Model file for the job. Use its own axes, mm. A direction names the side the tool comes from. Round coordinates to 2 decimals unless told otherwise and drop trailing zeros. Write each loop counter-clockwise with the first axis right and the second up, starting at its lowest first coordinate (ties: lowest second). Pieces come first, ordered by that corner, then holes.
```python
from build123d import *

# Parameters (mm, degrees)
F0_R     = 3.9
F1_DEPTH = 25
F0_R_2   = 6
F2_DEPTH = 5
F3_SIZE2 = 3
F3_SIZE  = 0.3


with BuildPart() as f1:
    # F0 (on Front) → F1 (new body)
    with BuildSketch(Plane.XZ):
        Circle(F0_R)
    extrude(amount=F1_DEPTH)

    # F0 (on Front) → F2 (join)
    with BuildSketch(Plane.XZ):
        Circle(F0_R_2)
        Circle(F0_R, mode=Mode.SUBTRACT)
    extrude(amount=F2_DEPTH)

    # F3
    f3_edges = [f1.edges().sort_by_distance(p)[0] for p in [
        (-3.9, -25, 0),
    ]]
    f3_side = f1.faces().sort_by_distance((0, -25, 0))[0]
    chamfer(f3_edges, length=F3_SIZE, length2=F3_SIZE2, reference=f3_side)


solid = f1.part
```
1) Cut at A-A on x = 0. List the corners of the cut face in (y, z), and give its area (3 significant figures).
2) Wall check: probe 1 along Y at (x, z) = (4.25, 3.5); probe 2 along X at (y, z) = (-4.25, 0.25); probe 3 along Z at (x, y) = (-2.25, -5.5). Give the ranges that are in metal, low to high.
3) Cut at B-B on z = 0. List the corners of the cut face in (x, y), and give its area (3 significant figures).
4) Cut at C-C on y = -16.5. List the corners of the cut face in (x, z).
5) Flat gauge pins, fed straight in: pin 1 Ø3 at (x, y) = (0, -12) entering from -Z; pin 2 Ø3 at (x, y) = (-4.5, -19) entering from -Z; pin 3 Ø2 at (x, y) = (-2, -14) entering from -Z. Where does each tip first touch, or does it go through?
6) Which spindle directions (+Z, -Z, +X, -X, +Y, -Y) get a long thin tool onto all of the face, cutting with end or side? Do faces 1 (the face through (0, 0, 0)), 2 (the face through (-2.87, -13.38, 2.64)). Say none if no direction does.
7) Cut at D-D on y = -3.5. List the corners of the cut face in (x, z), and give its area (3 significant figures).
Result sheet:
1. outline: (-25, -3.6) - (-22, -3.9) - (-5, -3.9) - (-5, -6) - (0, -6) - (0, 6) - (-5, 6) - (-5, 3.9) - (-22, 3.9) - (-25, 3.6) - close
1. area: 215 mm2
2. probe 1: y = -5 to 0
2. probe 2: x = -5.99 to 5.99
2. probe 3: z = -3.19 to 3.19
3. outline: (-6, -5) - (-3.9, -5) - (-3.9, -22) - (-3.6, -25) - (3.6, -25) - (3.9, -22) - (3.9, -5) - (6, -5) - (6, 0) - (-6, 0) - close
3. area: 215 mm2
4. outline: circle Ø7.8 at (0, 0)
5. pin 1: stops at z = -3.9
5. pin 2: stops at z = -2.49
5. pin 3: stops at z = -3.77
6. face 1: +Z, -Z, +X, -X, +Y
6. face 2: -Y
7. outline: circle Ø12 at (0, 0)
7. area: 113 mm2
